from build123d import *

# Parameters (mm, degrees)
SKETCH1_W           = 2000
SKETCH1_H           = 2000
SKETCH1_W_2         = 1900
SKETCH1_H_2         = 1900
SKETCH1_H_3         = 50
BOSS_EXTRUDE1_DEPTH = 300
SKETCH2_W           = 2000
SKETCH2_H           = 2000
BOSS_EXTRUDE2_DEPTH = 50


with BuildPart() as part:
    # Sketch1 → Boss-Extrude1 (new body)
    with BuildSketch(Plane.XY):
        Rectangle(SKETCH1_W, SKETCH1_H)
        Rectangle(SKETCH1_W_2, SKETCH1_H_2, mode=Mode.SUBTRACT)
        with Locations((0, 625)):
            Rectangle(SKETCH1_W_2, SKETCH1_H_3)
        with Locations((0, 274.988)):
            Rectangle(SKETCH1_W_2, SKETCH1_H_3)
        with Locations((0, -75.024)):
            Rectangle(SKETCH1_W_2, SKETCH1_H_3)
        with Locations((0, -425.036)):
            Rectangle(SKETCH1_W_2, SKETCH1_H_3)
        with Locations((0, -775.048)):
            Rectangle(SKETCH1_W_2, SKETCH1_H_3)
    extrude(amount=BOSS_EXTRUDE1_DEPTH)

    # Sketch2 → Boss-Extrude2 (add)
    with BuildSketch(Plane.XY.offset(300)):
        Rectangle(SKETCH2_W, SKETCH2_H)
    extrude(amount=BOSS_EXTRUDE2_DEPTH)


solid = part.part
For this review, take the finished solid that the model builds, in its own axes (mm). A direction names the side the tool comes from. Round coordinates to 2 decimals unless told otherwise and drop trailing zeros. Order: outer loops, then holes, each group sorted by start corner. A loop starts at its lowest first (then second) coordinate and runs counter-clockwise, first axis right, second up. Notation, with made-up numbers: M 14,-21 L 42,-21 A19 cw 42,-7 Z; hole C 53,-20.5 d2. An arc over 180 degrees is marked long. Use a Markdown table: item, result. Add a question column.
Item 1: Tool access review of faces 5 (the flat face through (-1000, -14, 173)), 6 (the flat face through (-13, -950, 148)): name each direction out of +Z, -Z, +X, -X, +Y, -Y from which nothing blocks a thin tool from reaching the whole face with its end or side.
Item 2: Mouldability with a two-part tool opening along Y and no side actions: class faces 1 (the flat face through (-950, 448, 148)), 2 (the flat face through (-5, -69, 0)), 3 (the flat face through (-950, -876, 148)), 4 (the flat face through (-14, 1000, 173)) as released by +Y, released by -Y, zero draft, split by the parting line, or undercut.
Item 3: To check wall thickness, follow line 1 along X through (y, z) = (53.5, 204); line 2 along Z through (x, y) = (379.5, 718). State the ranges of each line that lie inside material, in increasing order.
Item 4: Add section B-B, the plane y = -825.5. Give the boundary of the cut face in (x, z), then the cut area to 3 significant figures.
Item 5: Add section A-A, the plane z = 269. Give the boundary of the cut face in (x, y), then the cut area to 3 significant figures.
Item 6: Add section C-C, the plane x = 163. Give the boundary of the cut face in (y, z), then the cut area to 3 significant figures.
Geometry results:
| question | item | result |
|---|---|---|
| 1 | face 5 | +Z, -Z, -X, +Y, -Y |
| 1 | face 6 | -Z |
| 2 | face 1 | undercut |
| 2 | face 2 | zero draft |
| 2 | face 3 | undercut |
| 2 | face 4 | released by +Y |
| 3 | line 1 | x = -1000 to -950, 950 to 1000 |
| 3 | line 2 | z = 300 to 350 |
| 4 | outline | M -1000,0 L -950,0 L -950,300 L 950,300 L 950,0 L 1000,0 L 1000,350 L -1000,350 Z |
| 4 | area | 130,000 mm² |
| 5 | outline | M -1000,-1000 L 1000,-1000 L 1000,1000 L -1000,1000 Z; hole M -950,-950 L 950,-950 L 950,-800.05 L -950,-800.05 Z; hole M -950,-750.05 L 950,-750.05 L 950,-450.04 L -950,-450.04 Z; hole M -950,-400.04 L 950,-400.04 L 950,-100.02 L -950,-100.02 Z; hole M -950,-50.02 L 950,-50.02 L 950,249.99 L -950,249.99 Z; hole M -950,299.99 L 950,299.99 L 950,600 L -950,600 Z; hole M -950,650 L 950,650 L 950,950 L -950,950 Z |
| 5 | area | 865,000 mm² |
| 6 | outline | M -1000,0 L -950,0 L -950,300 L -800.05,300 L -800.05,0 L -750.05,0 L -750.05,300 L -450.04,300 L -450.04,0 L -400.04,0 L -400.04,300 L -100.02,300 L -100.02,0 L -50.02,0 L -50.02,300 L 249.99,300 L 249.99,0 L 299.99,0 L 299.99,300 L 600,300 L 600,0 L 650,0 L 650,300 L 950,300 L 950,0 L 1000,0 L 1000,350 L -1000,350 Z |
| 6 | area | 205,000 mm² |
